Check sheet for the modelled part. Datum: model origin and axes. Units: mm. Give positions to 0.01 mm unless a question says otherwise; leave off trailing zeros. Loops run counter-clockwise (first coordinate to the right, second up) from the corner with the lowest first, then second, coordinate; pieces in that order, holes last. Notation, with made-up numbers: M 81,-5 L 134,-5 A17 cw 134,23 Z; hole C 1,57 d6. An arc over 180 degrees is marked long. Use one line per item in the form item = value.
Autodesk Inventor part; units mm, degrees
ref_plane "YZ Plane" through (0, 0, 0) normal (1, 0, 0) x (0, 1, 0)
ref_plane "XZ Plane" through (0, 0, 0) normal (0, 1, 0) x (-1, 0, 0)
ref_plane "XY Plane" through (0, 0, 0) normal (0, 0, 1) x (1, 0, 0)
sketch "Sketch2" plane through (0, 0, 0) normal (0, 1, 0) x (-1, 0, 0)
  line L0 (-89, 99) -> (89, 99)
  line L1 (89, 99) -> (89, -99)
  line L2 (89, -99) -> (-89, -99)
  line L3 (-89, -99) -> (-89, 99)
  line L4 (-89, 99) -> (89, -99) construction
  line L5 (89, 99) -> (-89, -99) construction
  line L6 (-89, 99) -> (89, 99)
  line L7 (89, 99) -> (89, -85)
  line L8 (89, -85) -> (-89, -85)
  line L9 (-89, -85) -> (-89, 99)
  line L10 (-4.5, 99) -> (-89, 99)
  line L11 (-89, 99) -> (-89, 46)
  line L12 (-89, 46) -> (-4.5, 46)
  line L13 (-4.5, 46) -> (-4.5, 99)
  line L14 (4.5, 99) -> (89, 99)
  line L15 (89, 99) -> (89, 46)
  line L16 (89, 46) -> (4.5, 46)
  line L17 (4.5, 46) -> (4.5, 99)
  line L18 (22.5, 77.5) -> (22.5, 66.5)
  line L19 (16.5, 66.5) -> (16.5, 77.5)
  line L20 (-22.5, 66.5) -> (-22.5, 77.5)
  line L21 (-16.5, 77.5) -> (-16.5, 66.5)
  line L22 (-22.5, 99) -> (-16.5, 99)
  line L23 (-16.5, 99) -> (-16.5, 46)
  line L24 (-16.5, 46) -> (-22.5, 46)
  line L25 (-22.5, 46) -> (-22.5, 99)
  line L26 (16.5, 99) -> (22.5, 99)
  line L27 (22.5, 99) -> (22.5, 46)
  line L28 (22.5, 46) -> (16.5, 46)
  line L29 (16.5, 46) -> (16.5, 99)
  line L30 (-89, 99) -> (89, 99)
  line L31 (89, 99) -> (89, 98)
  line L32 (89, 98) -> (-89, 98)
  line L33 (-89, 98) -> (-89, 99)
  line L34 (89, -85) -> (73, -85)
  line L35 (73, -85) -> (73, -68)
  line L36 (73, -68) -> (89, -68)
  line L37 (89, -68) -> (89, -85)
  line L38 (-89, -85) -> (-73, -85)
  line L39 (-73, -85) -> (-73, -68)
  line L40 (-73, -68) -> (-89, -68)
  line L41 (-89, -68) -> (-89, -85)
  point P0 (0, 0)
  point P1 (4.5, 99)
  point P2 (-4.5, 99)
  point P3 (-89, 46)
  point P4 (89, 46)
  point P5 (4.5, 98)
  point P6 (-4.5, 98)
  point P7 (-16.5, 98)
  point P8 (-22.5, 98)
  point P9 (22.5, 98)
  point P10 (16.5, 98)
  point P11 (73, -85)
  dimension "d8" = 178
  dimension "d9" = 198
  dimension "d10" = 14
  dimension "d11" = 84.5
  dimension "d12" = 53
  dimension "d13" = 84.5
  dimension "d14" = 53
  dimension "d17" = 9
  dimension "d18" = 1
  dimension "d19" = 16
  dimension "d20" = 17
  dimension "d21" = 16
  dimension "d22" = 17
extrude "Extrusion2" add sketch "Sketch2" along normal blind 3 contours L32 L23 L21 L12 L25 L20 | L12 L13 L32 L17 L16 L1 L36 L35 L8 L39 L40 L3 | L32 L27 L18 L16 L29 L19
equation "\"d11\" = d13"
properties part number "base" material "Aluminum 6061-AHC"
1) Section check D-D (x = 78). Record the cut outline in (y, z).
Evaluation:
outline = M 0,-68 L 3,-68 L 3,46 L 0,46 Z
2) Section check C-C (x = -54). Record the cut outline in (y, z).
Evaluation:
outline = M 0,-85 L 3,-85 L 3,46 L 0,46 Z
3) Section check A-A (z = 61). Record the cut outline in (x, y), then the cut area to 3 significant figures.
Evaluation:
outline = M -22.5,0 L -16.5,0 L -16.5,3 L -22.5,3 Z; M -4.5,0 L 4.5,0 L 4.5,3 L -4.5,3 Z; M 16.5,0 L 22.5,0 L 22.5,3 L 16.5,3 Z
area = 63.0 mm^2
4) Release check for a two-part mould opening along Y. For faces 1 (the face through (1, 3, -13)), 2 (the face through (1, 0, -13)) record: pulls with the +Y half, pulls with the -Y half, needs draft (parallel to the pull), parting line crosses it, or undercut.
Evaluation:
face_1 = pulls with the +Y half
face_2 = pulls with the -Y half
5) Depth check by flat-ended pin: pin 1 Ø1.5 at (x, y) = (10.5, 2) entering from +Z; pin 2 Ø0.9 at (x, y) = (84.5, 1) entering from -Z; pin 3 Ø3 at (x, z) = (38.5, -16.5) entering from -Y; pin 4 Ø0.9 at (y, z) = (1.5, -80.5) entering from +X. Enter the tip coordinate at first touch or a pass-through.
Evaluation:
pin_1 = 46
pin_2 = -68
pin_3 = 0
pin_4 = 73
6) Section check B-B (y = 1.55). Record the cut outline in (x, z).
Evaluation:
outline = M -89,-68 L -73,-68 L -73,-85 L 73,-85 L 73,-68 L 89,-68 L 89,46 L 22.5,46 L 22.5,98 L 16.5,98 L 16.5,46 L 4.5,46 L 4.5,98 L -4.5,98 L -4.5,46 L -16.5,46 L -16.5,98 L -22.5,98 L -22.5,46 L -89,46 Z
7) Scan lines: line 1 (X direction, y = 0.5, z = 51.5); line 2 (Z direction, x = 35, y = 2.1); line 3 (X direction, y = 0.2, z = -72.5). Record each from-to range of solid material in increasing order.
Evaluation:
line_1 = -22.5 to -16.5, -4.5 to 4.5, 16.5 to 22.5
line_2 = -85 to 46
line_3 = -73 to 73
